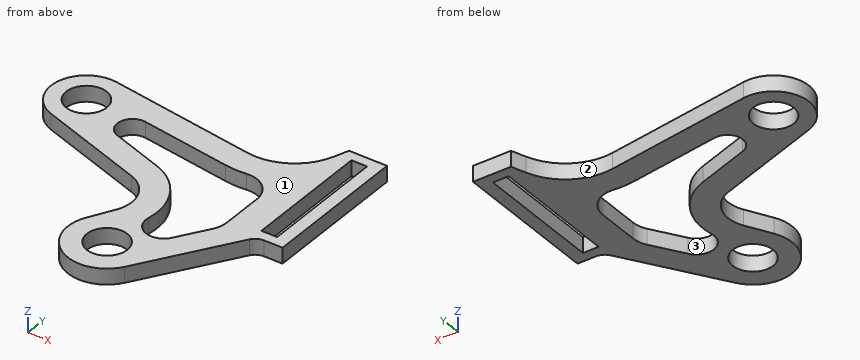
from build123d import *

# Parameters (mm, degrees)
SKETCH1_R           = 8
SKETCH1_W           = 6.2
SKETCH1_H           = 50
BOSS_EXTRUDE1_DEPTH = 6.2


with BuildPart() as part:
    # Sketch1 → Boss-Extrude1 (new body)
    with BuildSketch(Plane.XY):
        with BuildLine():
            Line((31.036127447, 82.458954329), (33, 88))
            Line((33, 88), (48, 88))
            Line((48, 88), (48, 30))
            Line((48, 30), (40.674945208, 30))
            ThreePointArc((40.674945208, 30), (38.288993634, 29.393999896), (36.481396821, 27.722894035))
            Line((36.481396821, 27.722894035), (13, -8.440971508))
            ThreePointArc((13, -8.440971508), (-7.975484523, -13.290660128), (-13.564659966, 7.5))
            Line((-13.564659966, 7.5), (-8.363522167, 16.906888758))
            ThreePointArc((-8.363522167, 16.906888758), (-7.61652309, 27.889035615), (-15.561762323, 35.507351095))
            Line((-15.561762323, 35.507351095), (-57.5, 49.742926416))
            ThreePointArc((-57.5, 49.742926416), (-66.602374097, 66.312916983), (-50.9, 76.841603953))
            Line((-50.9, 76.841603953), (7, 68.057217374))
            ThreePointArc((7, 68.057217374), (21.607393242, 70.936561685), (31.036127447, 82.458954329))
        make_face()
        with Locations(Location((-53, 63, 0), (0, 0, 180))):
            Circle(SKETCH1_R, mode=Mode.SUBTRACT)
        with Locations(Location((0, 0, 0), (0, 0, 180))):
            Circle(SKETCH1_R, mode=Mode.SUBTRACT)
        with Locations((39.9, 59)):
            Rectangle(SKETCH1_W, SKETCH1_H, mode=Mode.SUBTRACT)
        with BuildLine():
            Line((-30.073264159, 63.567409295), (5.5, 58.170357408))
            ThreePointArc((5.5, 58.170357408), (9.685179801, 57.814216157), (13.880952381, 58.009303341))
            ThreePointArc((13.880952381, 58.009303341), (21.663689812, 55.528335414), (25, 48.072113978))
            Line((25, 48.072113978), (25, 31.364873077))
            ThreePointArc((25, 31.364873077), (24.588299321, 28.525063906), (23.387096774, 25.919085008))
            Line((23.387096774, 25.919085008), (15.641533812, 13.990088635))
            ThreePointArc((15.641533812, 13.990088635), (7.184832002, 11.297220659), (2.884689445, 19.060990196))
            ThreePointArc((2.884689445, 19.060990196), (0.088285739, 34.851646077), (-12.347476609, 44.976689369))
            Line((-12.347476609, 44.976689369), (-32.901835588, 51.95369035))
            ThreePointArc((-32.901835588, 51.95369035), (-36.802853058, 59.055114879), (-30.073264159, 63.567409295))
        make_face(mode=Mode.SUBTRACT)
    extrude(amount=BOSS_EXTRUDE1_DEPTH)


solid = part.part
Design review of the part built by this model. Coordinates are the model's own, in mm. Face numbers are marked on the shaded views. Coordinates: 2 decimals unless noted, no trailing zeros. Order: outer loops, then holes, each group sorted by start corner. A loop starts at its lowest first (then second) coordinate and runs counter-clockwise, first axis right, second up. Notation, with made-up numbers: (71.5, 27) -> (121.5, 27) arc R15 ccw to (121.5, 43) -> close; hole circle Ø5 at (26.5, -23.5). An arc over 180 degrees is marked (long way). One line per item, written item: value.
1) We need section B-B, the plane y = 75. Give the boundary of the cut face in (x, z).
Output values:
outline: (-60.21, 0) -> (-38.76, 0) -> (-38.76, 6.2) -> (-60.21, 6.2) -> close; (26.57, 0) -> (36.8, 0) -> (36.8, 6.2) -> (26.57, 6.2) -> close; (43, 0) -> (48, 0) -> (48, 6.2) -> (43, 6.2) -> close
2) We need section A-A, the plane x = -17. Give the boundary of the cut face in (y, z), then the cut area to 3 significant figures.
Output values:
outline: (36, 0) -> (46.56, 0) -> (46.56, 6.2) -> (36, 6.2) -> close; (61.58, 0) -> (71.7, 0) -> (71.7, 6.2) -> (61.58, 6.2) -> close
area: 128 mm2
3) To check wall thickness, follow probe 1 along Y at (x, z) = (4.5, 1); probe 2 along Y at (x, z) = (0, 2); probe 3 along X at (y, z) = (34.5, 0.5). State the ranges of each line that lie inside material, in increasing order. Write a range as [from, to].
Output values:
probe 1: y = [-14.83, -6.61], [6.61, 13.2], [58.32, 68.44]
probe 2: y = [-15.5, -8], [8, 35], [59, 69.12]
probe 3: x = [-13.32, 0.29], [25, 36.8], [43, 48]
4) We need section D-D, the plane y = 0. Give the boundary of the cut face in (x, z).
Output values:
outline: (-15.5, 0) -> (-8, 0) -> (-8, 6.2) -> (-15.5, 6.2) -> close; (8, 0) -> (18.48, 0) -> (18.48, 6.2) -> (8, 6.2) -> close
5) Clearance check with flat-ended pins moving along their axes: P1, Ø2, axis at y = 34, z = 5.5, coming from the -X side; P2, Ø2, axis at x = 10, z = 2, coming from the +Y side. State where each tip first meets the part, or that it passes through.
Output values:
P1: stops at x = -14.29
P2: stops at y = 67.85
6) We need section C-C, the plane z = 3. Count the separate pieces of the cut face and the enclosed holes in it, then the cut area to 3 significant figures.
Output values:
separate pieces: 1
enclosed holes: 4
area: 3,660 mm2
7) Draft analysis for pull direction Y (two halves, no side actions). For the marked faces 1, 2 and 3, state which applies: +Y half, -Y half, draft (parallel to the pull), parting line (faces both ways), or undercut.
Output values:
face 1: draft
face 2: +Y half
face 3: undercut
